Autodesk Inventor part; units mm, degrees
ref_plane "YZ Plane" through (0, 0, 0) normal (1, 0, 0) x (0, 1, 0)
ref_plane "XZ Plane" through (0, 0, 0) normal (0, 1, 0) x (-1, 0, 0)
ref_plane "XY Plane" through (0, 0, 0) normal (0, 0, 1) x (1, 0, 0)
sketch "Sketch1" plane through (0, 0, 0) normal (0, 1, 0) x (-1, 0, 0)
  circle A0 centre (0, 0) radius 2.5
  dimension "d0" = 5
extrude "Extrusion1" add sketch "Sketch1" along normal blind 20
sketch "Sketch2" plane through (0, 20, 0) normal (0, 1, 0) x (1, 0, 0)
  circle A0 centre (0, 0) radius 2.5
  circle A1 centre (0, 0) radius 4.25
  dimension "d3" = 8.5
extrude "Extrusion2" add sketch "Sketch2" along normal blind 5 contours A0 | A1
sketch "Sketch3" plane through (0, 25, 0) normal (0, 1, 0) x (1, 0, 0)
  circle A0 centre (0, 0) radius 4.25
  line L0 (0, 2.3094) -> (2, 1.1547)
  line L1 (2, 1.1547) -> (2, -1.1547)
  line L2 (2, -1.1547) -> (0, -2.3094)
  line L3 (0, -2.3094) -> (-2, -1.1547)
  line L4 (-2, -1.1547) -> (-2, 1.1547)
  line L5 (-2, 1.1547) -> (0, 2.3094)
  dimension "d6" = 2
extrude "Extrusion3" cut sketch "Sketch3" against normal blind 3.2 contours L0 L1 L2 L3 L4 L5
thread "Thread1"
chamfer "Chamfer1" distance 0.25 angle 45 1 edges at (2.5, 0, 0)
properties part number "M5x22SHCS" material "Stainless Steel"
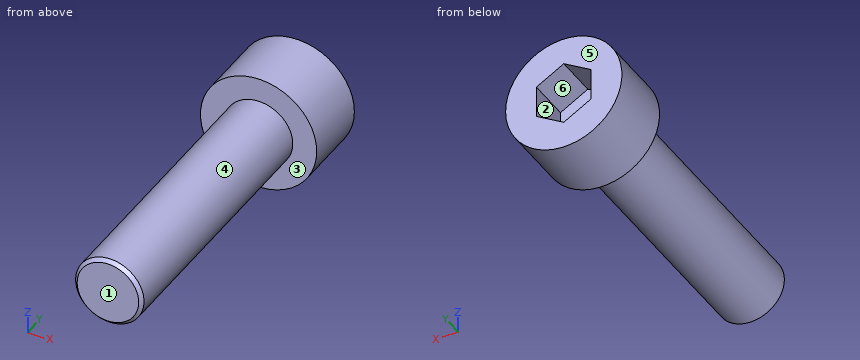
For this review, take the finished solid that the model builds, in its own axes (mm). Face numbers are marked on the shaded views. A direction names the side the tool comes from. Coordinates: 2 decimals unless noted, no trailing zeros. Loops run counter-clockwise (first coordinate to the right, second up) from the corner with the lowest first, then second, coordinate; pieces in that order, holes last.
1. Add section A-A, the plane y = 22.5. Give the boundary of the cut face in (x, z).
2. Mouldability with a two-part tool opening along X and no side actions: class the marked faces 4, 5 and 6 as +X half, -X half, draft (parallel to the pull), parting line (faces both ways), or undercut.
3. Add section D-D, the plane x = 3. Give the boundary of the cut face in (y, z), then the cut area to 3 significant figures.
4. For the marked faces 1, 2 and 3, list the 3-axis set-ups (+Z, -Z, +X, -X, +Y, -Y) from which the entire face can be reached by the end or side of a thin tool; tool diameter is ignored.
5. Insertion check: P1, Ø1.8, axis at y = 24, z = 0.5, coming from the +X side; P2, Ø3, axis at y = 21, z = 2.5, coming from the +X side; P3, Ø3, axis at y = 3.5, z = -3, coming from the +X side; P4, Ø2, axis at y = 9, z = -1, coming from the -X side. Each pin has a flat end and moves straight along its axis. Give the tip position at first contact, or say it passes through.
6. For line 1 (Y direction, x = -3.25, z = 2.25); line 2 (Y direction, x = 1, z = 0.25); line 3 (Z direction, x = 1.5, y = 3), list the stretches that pass through material, from the lowest coordinate up.
7. Add section C-C, the plane y = 11.25. Give the boundary of the cut face in (x, z).
8. Add section B-B, the plane z = 0. Give the boundary of the cut face in (x, y).
Result:
1. outline: circle Ø8.5 at (0, 0); hole (-2, -1.15) - (0, -2.31) - (2, -1.15) - (2, 1.15) - (0, 2.31) - (-2, 1.15) - close
2. face 4: parting line
2. face 5: draft
2. face 6: undercut
3. outline: (20, -3.01) - (25, -3.01) - (25, 3.01) - (20, 3.01) - close
3. area: 30.1 mm2
4. face 1: +Z, -Z, +X, -X, -Y
4. face 2: +Y
4. face 3: -Y
5. P1: stops at x = 4.25
5. P2: stops at x = 4.13
5. P3: stops at x = 2
5. P4: stops at x = -2.5
6. line 1: y = 20 to 25
6. line 2: y = 0 to 21.8
6. line 3: z = -2 to 2
7. outline: circle Ø5 at (0, 0)
8. outline: (-4.25, 20) - (-2.5, 20) - (-2.5, 0.25) - (-2.25, 0) - (2.25, 0) - (2.5, 0.25) - (2.5, 20) - (4.25, 20) - (4.25, 25) - (2, 25) - (2, 21.8) - (-2, 21.8) - (-2, 25) - (-4.25, 25) - close
